```python
from build123d import *

# Parameters (mm, degrees)
SKETCH1_W           = 44
SKETCH1_H           = 23
BOSS_EXTRUDE1_DEPTH = 2
SKETCH2_W           = 3.9
SKETCH2_H           = 8.6
SKETCH2_W_2         = 7
SKETCH2_H_2         = 1.5
SKETCH2_W_3         = 20.7
SKETCH2_H_3         = 2
CUT_EXTRUDE1_DEPTH  = 2
SKETCH4_W           = 8
SKETCH4_H           = 2
BOSS_EXTRUDE2_DEPTH = 6


with BuildPart() as part:
    # Sketch1 → Boss-Extrude1 (new body)
    with BuildSketch(Plane.XY):
        Rectangle(SKETCH1_W, SKETCH1_H)
    extrude(amount=BOSS_EXTRUDE1_DEPTH)

    # Sketch2 → Cut-Extrude1 (cut)
    with BuildSketch(Plane.XY.offset(2)):
        with Locations((-18.05, -5.2)):
            Rectangle(SKETCH2_W, SKETCH2_H)
        with Locations((12.4, -8.75)):
            Rectangle(SKETCH2_W_2, SKETCH2_H_2)
        with Locations((-1.65, 6.7)):
            Rectangle(SKETCH2_W_3, SKETCH2_H_3)
    extrude(amount=-CUT_EXTRUDE1_DEPTH, mode=Mode.SUBTRACT)

    # Sketch4 → Boss-Extrude2 (add)
    with BuildSketch(Plane.XY.offset(2)):
        with Locations((-11, -10.5)):
            Rectangle(SKETCH4_W, SKETCH4_H)
        with Locations((0, -10.5)):
            Rectangle(SKETCH4_W, SKETCH4_H)
        with Locations((11, -10.5)):
            Rectangle(SKETCH4_W, SKETCH4_H)
    extrude(amount=BOSS_EXTRUDE2_DEPTH)


solid = part.part
```
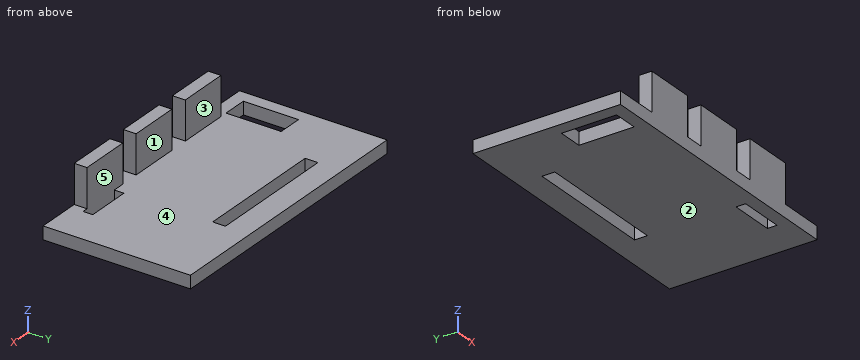
The model under review builds one solid part; all positions refer to its coordinate system, in mm. Face numbers are marked on the shaded views. A direction names the side the tool comes from. Coordinates: 2 decimals unless noted, no trailing zeros. Write each loop counter-clockwise with the first axis right and the second up, starting at its lowest first coordinate (ties: lowest second). Pieces come first, ordered by that corner, then holes. Notation, with made-up numbers: (25.25, -23) - (60.25, -23) arc R22 cw to (60.25, 4) - close; hole circle Ø1 at (-25, -11). An arc over 180 degrees is marked (long way). Answer in a Markdown table with one row per item. Add a question column.
Q1. Consider section D-D on y = 8.75. Give the boundary of the cut face in (x, z).
Q2. Consider section C-C on x = 3.5. Give the boundary of the cut face in (y, z), then the cut area to 3 significant figures.
Q3. For the marked faces 1 and 2, list the 3-axis set-ups (+Z, -Z, +X, -X, +Y, -Y) from which the entire face can be reached by the end or side of a thin tool; tool diameter is ignored.
Q4. Draft analysis for pull direction Y (two halves, no side actions). For the marked faces 3, 4 and 5, state which applies: +Y half, -Y half, draft (parallel to the pull), parting line (faces both ways), or undercut.
Q5. Consider section B-B on x = -18. Give the boundary of the cut face in (y, z).
Q6. Clearance check with flat-ended pins moving along their axes: pin 1 (3 mm diameter, centred on x = -11.5, z = 4.5, fed in from +Y); pin 2 (7 mm diameter, centred on x = -7.5, y = 5, fed in from +Z); pin 3 (1.5 mm diameter, centred on y = -7.5, z = 7, fed in from -X); pin 4 (2 mm diameter, centred on y = -10, z = 4, fed in from +X). State where each tip first meets the part, or that it passes through.
Q7. To check wall thickness, follow line 1 along Z through (x, y) = (-12.5, 1.25); line 2 along Y through (x, z) = (-17.5, 0.75); line 3 along Y through (x, z) = (8.5, 1). State the ranges of each line that lie inside material, in increasing order. Write a range as from..to.
Q8. Consider section A-A on y = -3. Give the boundary of the cut face in (x, z).
Answers below:
| question | item | result |
|---|---|---|
| 1 | outline | (-22, 0) - (22, 0) - (22, 2) - (-22, 2) - close |
| 2 | outline | (-11.5, 0) - (5.7, 0) - (5.7, 2) - (-9.5, 2) - (-9.5, 8) - (-11.5, 8) - close; (7.7, 0) - (11.5, 0) - (11.5, 2) - (7.7, 2) - close |
| 2 | area | 54.0 mm² |
| 3 | face 1 | +Z, +X, -X, +Y |
| 3 | face 2 | -Z, +X, -X, +Y, -Y |
| 4 | face 3 | +Y half |
| 4 | face 4 | draft |
| 4 | face 5 | undercut |
| 5 | outline | (-11.5, 0) - (-9.5, 0) - (-9.5, 2) - (-11.5, 2) - close; (-0.9, 0) - (11.5, 0) - (11.5, 2) - (-0.9, 2) - close |
| 6 | pin 1 | y = -9.5 |
| 6 | pin 2 | z = 2 |
| 6 | pin 3 | through |
| 6 | pin 4 | x = 15 |
| 7 | line 1 | 0..2 |
| 7 | line 2 | -11.5..-9.5, -0.9..11.5 |
| 7 | line 3 | -11.5..5.7, 7.7..11.5 |
| 8 | outline | (-22, 0) - (-20, 0) - (-20, 2) - (-22, 2) - close; (-16.1, 0) - (22, 0) - (22, 2) - (-16.1, 2) - close |
